Could you check a few things on this model? Use its own coordinates, in mm. Face numbers are marked on the shaded views. A direction names the side the tool comes from. Give positions to 0.01 mm unless a question says otherwise; leave off trailing zeros. Loops run counter-clockwise (first coordinate to the right, second up) from the corner with the lowest first, then second, coordinate; pieces in that order, holes last. Notation, with made-up numbers: (44.25, 3) - (53.25, 3) arc R15 cw to (53.25, 25) - close; hole circle Ø10 at (48, 70.5). An arc over 180 degrees is marked (long way). Use CSV: the item, a comma, the result in double quotes.
from build123d import *

# Parameters (mm, degrees)
SKETCH1_W           = 10
SKETCH1_H           = 15.5
SKETCH1_R           = 1.85
BOSS_EXTRUDE1_DEPTH = 0.55
SKETCH2_W           = 10
SKETCH2_H           = 9.25
BOSS_EXTRUDE2_DEPTH = 3.75
CHAMFER1_SIZE       = 4
CHAMFER1_SIZE_2     = 1
SKETCH3_W           = 1.3
SKETCH3_H           = 0.5
BOSS_EXTRUDE3_DEPTH = 13
CUT_EXTRUDE1_DEPTH  = 19.688231591


with BuildPart() as part:
    # Sketch1 → Boss-Extrude1 (new body)
    with BuildSketch(Plane(origin=(0, 0, 0), x_dir=(1, 0, 0), z_dir=(0, 1, 0))):
        with Locations((5, 7.75)):
            Rectangle(SKETCH1_W, SKETCH1_H)
        with Locations(Location((5, 12.75, 0), (0, 0, 270))):
            Circle(SKETCH1_R, mode=Mode.SUBTRACT)
    extrude(amount=BOSS_EXTRUDE1_DEPTH)

    # Sketch2 → Boss-Extrude2 (add)
    with BuildSketch(Plane(origin=(0, 0.55, 0), x_dir=(1, 0, 0), z_dir=(0, 1, 0))):
        with Locations((5, 4.625)):
            Rectangle(SKETCH2_W, SKETCH2_H)
    extrude(amount=BOSS_EXTRUDE2_DEPTH)

    # Chamfer1
    # the kernel refuses this chamfer: 4, 1 mm, written as the material it takes off along each edge
    with BuildSketch(Plane(origin=(20.388509999, 4.3, -9.25), x_dir=(0, -0.9999563942249224, -0.00933861064031752), z_dir=(-1, 0, 0))) as chamfer1_piece_1_section:
        Polygon((CHAMFER1_SIZE * 0.999956394225, CHAMFER1_SIZE * 0.00933861064032), (-CHAMFER1_SIZE_2 * 0.00933861064032, CHAMFER1_SIZE_2 * 0.999956394225), (0, 0), align=None)
    chamfer1_piece_1 = extrude(amount=30.777019998, mode=Mode.PRIVATE)
    chamfer1_piece_1 = split(chamfer1_piece_1, bisect_by=Plane(origin=(5, 0.55, -8.951597726), z_dir=(0, 1, 0)), keep=Keep.TOP, mode=Mode.PRIVATE)
    add(chamfer1_piece_1, mode=Mode.SUBTRACT)

    # Sketch3 → Boss-Extrude3 (add)
    with BuildSketch(Plane.XY):
        with Locations((2.5, 2.75)):
            Rectangle(SKETCH3_W, SKETCH3_H)
        with Locations((5, 2.75)):
            Rectangle(SKETCH3_W, SKETCH3_H)
        with Locations((7.5, 2.75)):
            Rectangle(SKETCH3_W, SKETCH3_H)
    extrude(amount=BOSS_EXTRUDE3_DEPTH)

    # Sketch4 → Cut-Extrude1 (cut, through all)
    with BuildSketch(Plane(origin=(0, 3, 0), x_dir=(1, 0, 0), z_dir=(0, 1, 0))):
        Polygon((1.85, -3.2), (2.15, -3.8), (2.15, -13), (1.85, -13), align=None)
        Polygon((4.35, -3.2), (4.65, -3.8), (4.65, -13), (4.35, -13), align=None)
        Polygon((6.85, -3.2), (7.15, -3.8), (7.15, -13), (6.85, -13), align=None)
        Polygon((3.15, -3.2), (2.85, -3.8), (2.85, -13), (3.15, -13), align=None)
        Polygon((5.65, -3.2), (5.35, -3.8), (5.35, -13), (5.65, -13), align=None)
        Polygon((8.15, -3.2), (7.85, -3.8), (7.85, -13), (8.15, -13), align=None)
    extrude(amount=-CUT_EXTRUDE1_DEPTH, mode=Mode.SUBTRACT)


solid = part.part
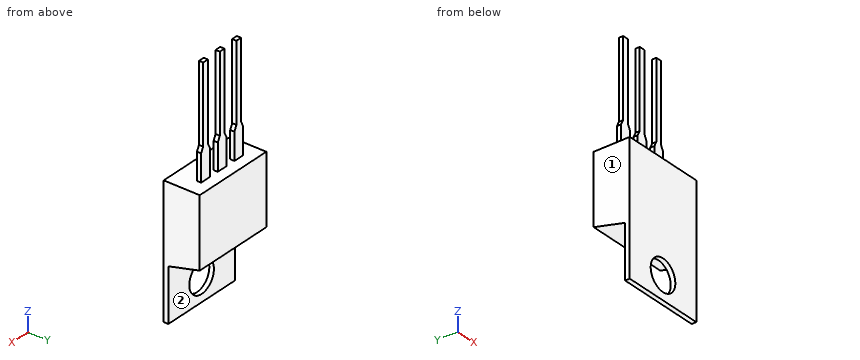
1) I need wall thicknesses on line 1 along X through (y, z) = (2.75, 9.25); line 2 along X through (y, z) = (0.3, -12.75); line 3 along Y through (x, z) = (7, -13.25). Which ranges of each line are inside material? Lowest first, please.
Answer below:
line 1,"x = 2.15 to 2.85, 4.65 to 5.35, 7.15 to 7.85"
line 2,"x = 0 to 3.15, 6.85 to 10"
line 3,"y = 0 to 0.55"
2) Suppose I cut it at C-C (z = -12.75). Please give me the cut outline in (x, y).
Answer below:
outline,"(0, 0) - (3.15, 0) - (3.15, 0.55) - (0, 0.55) - close; (6.85, 0) - (10, 0) - (10, 0.55) - (6.85, 0.55) - close"
3) Suppose I cut it at A-A (z = 7.5). Please give me the cut outline in (x, y).
Answer below:
outline,"(2.15, 2.5) - (2.85, 2.5) - (2.85, 3) - (2.15, 3) - close; (4.65, 2.5) - (5.35, 2.5) - (5.35, 3) - (4.65, 3) - close; (7.15, 2.5) - (7.85, 2.5) - (7.85, 3) - (7.15, 3) - close"
4) Suppose I cut it at B-B (x = 5). Please give me the cut outline in (y, z), plus the area to 3 significant figures.
Answer below:
outline,"(0, -15.5) - (0.55, -15.5) - (0.55, -14.6) - (0, -14.6) - close; (0, -10.9) - (0.55, -10.9) - (0.55, -9.19) - (4.3, -8.25) - (4.3, 0) - (3, 0) - (3, 13) - (2.5, 13) - (2.5, 0) - (0, 0) - close"
area,"45.7 mm2"
5) Which directions (+Z, -Z, +X, -X, +Y, -Y) give clear straight access to the entire face, cutting with the end or side of a thin tool? Please do the marked faces 1 and 2.
Answer below:
face 1,"+Z, -Z, -X, +Y, -Y"
face 2,"-Z, +X, -X, +Y"
6) Suppose I cut it at D-D (x = 6.5). Please give me the cut outline in (y, z), plus the area to 3 significant figures.
Answer below:
outline,"(0, -15.5) - (0.55, -15.5) - (0.55, -13.83) - (0, -13.83) - close; (0, -11.67) - (0.55, -11.67) - (0.55, -9.19) - (4.3, -8.25) - (4.3, 0) - (0, 0) - close"
area,"40.0 mm2"
7) I'm going to push flat-ended pins straight in: P1, Ø5, axis at x = 5.5, z = -13.5, coming from the +Y side; P2, Ø1, axis at x = 5, z = 9, coming from the +Y side; P3, Ø0.6, axis at y = 3, z = 2.5, coming from the +X side. Where does each tip first touch, or does it pass through?
Answer below:
P1,"stops at y = 0.55"
P2,"stops at y = 3"
P3,"stops at x = 8.15"
